from build123d import *

# Parameters (mm, degrees)
F0_R     = 9.525
F1_DEPTH = 9.525
F2_R     = 25.4
F3_DEPTH = 3.175
F4_R     = 6.35
F5_DEPTH = 12.7


# Not quite as in the source:
# - a length typed as a fraction of an inch, garbled in the dataset ("3 / 203.2 mm" for 3/8 in), is restored


with BuildPart() as f1:
    # F0 (on Front) → F1 (new body)
    with BuildSketch(Plane.XZ):
        Circle(F0_R)
    extrude(amount=F1_DEPTH)

    # F2 (on face) → F3 (join)
    with BuildSketch(Plane.XZ.offset(9.525)):
        Circle(F2_R)
    extrude(amount=-F3_DEPTH)

    # F4 (on face) → F5 (cut, symmetric)
    with BuildSketch(Plane.XZ.offset(9.525)):
        Circle(F4_R)
    extrude(amount=F5_DEPTH, both=True, mode=Mode.SUBTRACT)

    # F6: F1 across plane


with BuildPart() as f1_1:
    add(f1.part)
    add(f1.part.mirror(Plane.XZ))


solid = f1_1.part
Geometry: final body of the model. Coordinates: model frame, mm. A direction names the side the tool comes from. Coordinates: 2 decimals unless noted, no trailing zeros. Order: outer loops, then holes, each group sorted by start corner. A loop starts at its lowest first (then second) coordinate and runs counter-clockwise, first axis right, second up.
(1) Access query for faces 1 (the face through (-5.506, -7.96, -24.796)), 2 (the face through (11, -6.35, 0)). Directions: +Z, -Z, +X, -X, +Y, -Y. A direction counts if a zero-diameter tool reaches every point of the face in a straight line with its end or side. Return the directions, or none.
(2) Section query C-C (y = 5.5). Return the cut outline in (x, z) (3 decimals).
(3) Section query D-D (x = -11). Return the cut outline in (y, z) (3 decimals).
(4) Section query A-A (z = 0). Return the cut outline in (x, y) (3 decimals), plus the area to 3 significant figures.
(5) First-contact query: pin 1 (2 mm diameter, centred on y = -2, z = 9, fed in from +X); pin 2 (10 mm diameter, centred on y = 4.5, z = -7, fed in from -X); pin 3 (2 mm diameter, centred on y = 5.5, z = 8, fed in from +X). Flat tips, straight axial feed; report the tip coordinate or a pass-through.
(6) Section query B-B (x = 0). Return the cut outline in (y, z) (3 decimals), plus the area to 3 significant figures.
(7) Material intervals for probe 1 along Y at (x, z) = (11.5, -14.5) (3 decimals); probe 2 along Z at (x, y) = (0, -7), sorted ascending.
Solution:
1. face 1: +Y, -Y
1. face 2: none
2. outline: circle Ø19.05 at (0, 0); hole circle Ø12.7 at (0, 0)
3. outline: (-9.525, -22.895) - (-6.35, -22.895) - (-6.35, 22.895) - (-9.525, 22.895) - close; (6.35, -22.895) - (9.525, -22.895) - (9.525, 22.895) - (6.35, 22.895) - close
4. outline: (-25.4, -9.525) - (-6.35, -9.525) - (-6.35, 9.525) - (-25.4, 9.525) - (-25.4, 6.35) - (-9.525, 6.35) - (-9.525, -6.35) - (-25.4, -6.35) - close; (6.35, -9.525) - (25.4, -9.525) - (25.4, -6.35) - (9.525, -6.35) - (9.525, 6.35) - (25.4, 6.35) - (25.4, 9.525) - (6.35, 9.525) - close
4. area: 323 mm2
5. pin 1: stops at x = 5.17
5. pin 2: stops at x = -25.29
5. pin 3: stops at x = 24.28
6. outline: (-9.525, -25.4) - (-6.35, -25.4) - (-6.35, -9.525) - (6.35, -9.525) - (6.35, -25.4) - (9.525, -25.4) - (9.525, -6.35) - (-9.525, -6.35) - close; (-9.525, 6.35) - (9.525, 6.35) - (9.525, 25.4) - (6.35, 25.4) - (6.35, 9.525) - (-6.35, 9.525) - (-6.35, 25.4) - (-9.525, 25.4) - close
6. area: 323 mm2
7. probe 1: y = -9.525 to -6.35, 6.35 to 9.525
7. probe 2: z = -25.4 to -6.35, 6.35 to 25.4
